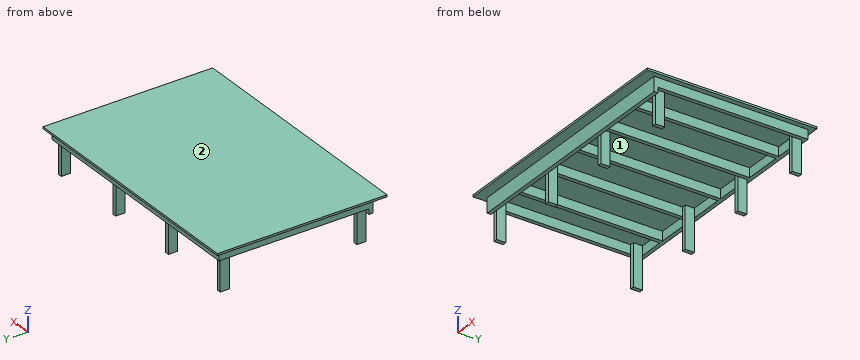
```python
from build123d import *

# Parameters (mm, degrees)
F0_W     = 2438.4
F0_H     = 914.4
F0_H_2   = 723.9
F1_DEPTH = 19.05
F2_W     = 2336.8
F2_H     = 1485.9
F2_W_2   = 279.4
F2_H_2   = 1409.7
F2_W_3   = 368.3
F2_W_4   = 317.5
F3_DEPTH = 88.9
F4_W     = 2336.8
F4_H     = 38.1
F5_DEPTH = 50.8
F6_W     = 38.1
F6_H     = 88.9
F7_DEPTH = 406.4


with BuildPart() as f1:
    # F0 (on Top) → F1 (new body)
    with BuildSketch(Plane.XY):
        with Locations((1219.2, -457.2)):
            Rectangle(F0_W, F0_H)
        with Locations((1219.2, -1276.35)):
            Rectangle(F0_W, F0_H_2)
    extrude(amount=F1_DEPTH)

    # F2 (on face) → F3 (join)
    with BuildSketch(Plane(origin=(0, 0, 0), x_dir=(1, 0, 0), z_dir=(0, 0, -1))):
        with Locations((1219.2, 793.75)):
            Rectangle(F2_W, F2_H)
        with Locations((228.6, 793.75)):
            Rectangle(F2_W_2, F2_H_2, mode=Mode.SUBTRACT)
        with Locations((590.55, 793.75)):
            Rectangle(F2_W_3, F2_H_2, mode=Mode.SUBTRACT)
        with Locations((996.95, 793.75)):
            Rectangle(F2_W_3, F2_H_2, mode=Mode.SUBTRACT)
        with Locations((1403.35, 793.75)):
            Rectangle(F2_W_3, F2_H_2, mode=Mode.SUBTRACT)
        with Locations((1809.75, 793.75)):
            Rectangle(F2_W_3, F2_H_2, mode=Mode.SUBTRACT)
        with Locations((2190.75, 793.75)):
            Rectangle(F2_W_4, F2_H_2, mode=Mode.SUBTRACT)
    extrude(amount=F3_DEPTH)

    # F4 (on face) → F5 (join)
    with BuildSketch(Plane(origin=(0, 0, -88.9), x_dir=(1, 0, 0), z_dir=(0, 0, -1))):
        with Locations((1219.2, 1517.65)):
            Rectangle(F4_W, F4_H)
    extrude(amount=F5_DEPTH)

    # F6 (on face) → F7 (join)
    with BuildSketch(Plane(origin=(0, 0, 0), x_dir=(1, 0, 0), z_dir=(0, 0, -1))):
        with Locations((107.95, 133.35)):
            Rectangle(F6_W, F6_H)
        with Locations((2330.45, 133.35)):
            Rectangle(F6_W, F6_H)
        with Locations((2330.45, 1454.15)):
            Rectangle(F6_W, F6_H)
        with Locations((107.95, 1454.15)):
            Rectangle(F6_W, F6_H)
        with Locations((831.85, 133.35)):
            Rectangle(F6_W, F6_H)
        with Locations((1568.45, 133.35)):
            Rectangle(F6_W, F6_H)
        with Locations((1568.45, 1454.15)):
            Rectangle(F6_W, F6_H)
        with Locations((831.85, 1454.15)):
            Rectangle(F6_W, F6_H)
    extrude(amount=F7_DEPTH)


solid = f1.part
```
Check sheet for the modelled part. Datum: model origin and axes. Units: mm. Face numbers are marked on the shaded views. Round coordinates to 2 decimals unless told otherwise and drop trailing zeros. Loops run counter-clockwise (first coordinate to the right, second up) from the corner with the lowest first, then second, coordinate; pieces in that order, holes last. Notation, with made-up numbers: (62, 65.5) - (69, 65.5) arc R38 cw to (69, 104.5) - close; hole circle Ø6 at (83, 27). An arc over 180 degrees is marked (long way). Answer as a JSON object with one key per item and string values. Group by question number.
Q1. Sectioned sample at B-B, the plane z = -372. Count the separate pieces of the cut face and the enclosed holes in it, plus the area to 3 significant figures.
Q2. Scan lines: line 1 along X through (y, z) = (-1457.5, -267); line 2 along Y through (x, z) = (1935.5, -63); line 3 along Y through (x, z) = (2321.5, -365). Record each from-to range of solid material in increasing order. Write a range as [from, to].
Q3. Sectioned sample at C-C, the plane x = 1414.5. Enter the section's corners in (y, z), plus the area to 3 significant figures.
Q4. Mould release check, pull along X, two halves, no side actions. Record for the marked faces 1 and 2: released by +X, released by -X, zero draft, split by the parting line, or undercut.
Q5. Gauge pin test, flat ends, axial feed: P1, Ø8, axis at y = -1250, z = -40.5, coming from the -X side; P2, Ø1.5, axis at x = 1830, y = -779.5, coming from the -Z side; P3, Ø19, axis at x = 2327, z = -320, coming from the +Y side. Record the tip position at first contact, or that the pin passes through.
Solution:
{
 "1": {"separate pieces": "8", "enclosed holes": "0", "area": "27,100 mm²"},
 "2": {"line 1": "x = [88.9, 127], [812.8, 850.9], [1549.4, 1587.5], [2311.4, 2349.5]", "line 2": "y = [-1536.7, -1498.6], [-88.9, -50.8]", "line 3": "y = [-1498.6, -1409.7], [-177.8, -88.9]"},
 "3": {"outline": "(-1638.3, 0) - (-1536.7, 0) - (-1536.7, -139.7) - (-1498.6, -139.7) - (-1498.6, 0) - (-88.9, 0) - (-88.9, -88.9) - (-50.8, -88.9) - (-50.8, 0) - (0, 0) - (0, 19.05) - (-1638.3, 19.05) - close", "area": "39,900 mm²"},
 "4": {"face 1": "undercut", "face 2": "zero draft"},
 "5": {"P1": "stops at x = 50.8", "P2": "stops at z = 0", "P3": "stops at y = -88.9"}
}
